```python
from build123d import *

# Parameters (mm, degrees)
SKETCH_R     = 1.5
PAD_DEPTH    = 2
PAD001_DEPTH = 34
CHAMFER_SIZE = 2
SKETCH002_R  = 1
PAD002_DEPTH = 5.5


with BuildPart() as part:
    # Sketch → Pad (new body)
    with BuildSketch(Plane.XY):
        with BuildLine():
            ThreePointArc((-9.697093, 1.874583), (-11, 0), (-9.697093, -1.874583))
            Line((-3, -4.365), (-9.697093, -1.874583))
            Line((3, -4.365), (-3, -4.365))
            Line((9.697093, -1.874583), (3, -4.365))
            ThreePointArc((9.697093, -1.874583), (11, 0), (9.697093, 1.874583))
            Line((3, 4.365), (9.697093, 1.874583))
            Line((-3, 4.365), (3, 4.365))
            Line((-9.697093, 1.874583), (-3, 4.365))
        make_face()
        with Locations((-9, 0)):
            Circle(SKETCH_R, mode=Mode.SUBTRACT)
        with Locations((9, 0)):
            Circle(SKETCH_R, mode=Mode.SUBTRACT)
    extrude(amount=PAD_DEPTH)

    # Sketch001 (on Face12 of Pad) → Pad001 (join)
    with BuildSketch(Plane.XY.offset(2)):
        Polygon((-3, 4.365), (-6.5, 1.5), (-6.5, -1.5), (-3, -4.365), (3, -4.365), (6.5, -1.5), (6.5, 1.5), (3, 4.365), align=None)
    extrude(amount=PAD001_DEPTH)

    # Chamfer
    chamfer_edges = [part.edges().sort_by_distance(p)[0] for p in [
        (6.5, 0, 36),
        (4.75, -2.9325, 36),
        (0, -4.365, 36),
        (-4.75, -2.9325, 36),
        (-6.5, 0, 36),
        (-4.75, 2.9325, 36),
        (0, 4.365, 36),
        (4.75, 2.9325, 36),
    ]]
    chamfer(chamfer_edges, length=CHAMFER_SIZE)

    # Sketch002 (on Face9 of Chamfer) → Pad002 (join)
    with BuildSketch(Plane.XY.offset(36)):
        Circle(SKETCH002_R)
    extrude(amount=PAD002_DEPTH)


solid = part.part
```
For this review, take the finished solid that the model builds, in its own axes (mm). A direction names the side the tool comes from. Give positions to 0.01 mm unless a question says otherwise; leave off trailing zeros. Write each loop counter-clockwise with the first axis right and the second up, starting at its lowest first coordinate (ties: lowest second). Pieces come first, ordered by that corner, then holes.
Item 1: Machinability: for faces 1 (the face through (-6.5, 0, 18)), 2 (the face through (4.73, -2.95, 17.78)), 3 (the face through (4.774, 2.912, 17.776)), which of the approach directions +Z, -Z, +X, -X, +Y, -Y give a long, thin tool a straight path to every point of the face, cutting with its end or side? Answer none if there is none.
Item 2: Take a section at A-A (z = 16.5). Give the boundary of the cut face in (x, y) (3 decimals), and give its area (3 significant figures).
Item 3: Wall thickness on probe 1 along X at (y, z) = (-1.5, 19); probe 2 along Z at (x, y) = (-2.5, 0); probe 3 along Y at (x, z) = (-9, 1.55): over which ranges is each line inside the solid? List them lowest first.
Item 4: Take a section at D-D (y = 2.75). Give the boundary of the cut face in (x, z) (3 decimals).
Item 5: Take a section at C-C (x = 9). Give the boundary of the cut face in (y, z), and give its area (3 significant figures).
Item 6: The part is to be moulded in two halves that separate along Y. For faces 4 (the face through (-10.5, 0.07, 0.99)), 5 (the face through (-4.083, 2.168, 35.014)), 6 (the face through (0, -4.365, 17)), say which applies: +Y half, -Y half, draft (parallel to the pull), parting line (faces both ways), or undercut.
Item 7: Insertion check: P1, Ø2, axis at x = 1.5, y = -1.5, coming from the -Z side; P2, Ø3.5, axis at y = -0.5, z = 16, coming from the +X side; P3, Ø3, axis at x = 3.5, y = 2, coming from the +Z side; P4, Ø3, axis at x = 5, z = 30.5, coming from the +Y side. Each pin has a flat end and moves straight along its axis. Give the tip position at first contact, or say it passes through.
Item 8: Take a section at B-B (x = 0). Give the boundary of the cut face in (y, z) (3 decimals), and give its area (3 significant figures).
Established:
1. face 1: +Z, -X, +Y, -Y
1. face 2: +Z, +X, -Y
1. face 3: +Z, +X, +Y
2. outline: (-6.5, -1.5) - (-3, -4.365) - (3, -4.365) - (6.5, -1.5) - (6.5, 1.5) - (3, 4.365) - (-3, 4.365) - (-6.5, 1.5) - close
2. area: 93.4 mm2
3. probe 1: x = -6.5 to 6.5
3. probe 2: z = 0 to 36
3. probe 3: y = -2.13 to -1.5, 1.5 to 2.13
4. outline: (-7.343, 0) - (7.343, 0) - (7.343, 2) - (4.973, 2) - (4.973, 34) - (2.423, 35.615) - (-2.423, 35.615) - (-4.973, 34) - (-4.973, 2) - (-7.343, 2) - close
5. outline: (-2.13, 0) - (-1.5, 0) - (-1.5, 2) - (-2.13, 2) - close; (1.5, 0) - (2.13, 0) - (2.13, 2) - (1.5, 2) - close
5. area: 2.54 mm2
6. face 4: undercut
6. face 5: +Y half
6. face 6: -Y half
7. P1: stops at z = 0
7. P2: stops at x = 6.5
7. P3: stops at z = 36
7. P4: stops at y = 3.96
8. outline: (-4.365, 0) - (4.365, 0) - (4.365, 34) - (2.365, 36) - (1, 36) - (1, 41.5) - (-1, 41.5) - (-1, 36) - (-2.365, 36) - (-4.365, 34) - close
8. area: 321 mm2
